```python
from build123d import *

# Parameters (mm, degrees)
F0_W     = 100
F0_H     = 100
F1_DEPTH = 15
F3_DEPTH = 25
F4_R     = 30
F5_DEPTH = 15.001
F6_W     = 20
F6_H     = 20
F7_DEPTH = 60
F8_W     = 80
F8_H     = 80
F9_DEPTH = 15.001


with BuildPart() as f1:
    # F0 (on Top) → F1 (new body)
    with BuildSketch(Plane.XY):
        Rectangle(F0_W, F0_H)
    extrude(amount=F1_DEPTH)

    # F2 (on face) → F3 (join)
    with BuildSketch(Plane.XY.offset(15)):
        Polygon((-30, -50), (-30, 30), (50, 30), (50, 50), (-50, 50), (-50, -50), align=None)
    extrude(amount=F3_DEPTH)

    # F4 (on face) → F5 (cut, through all)
    with BuildSketch(Plane.XY.offset(15)):
        with Locations((10, -10)):
            Circle(F4_R)
    extrude(amount=-F5_DEPTH, mode=Mode.SUBTRACT)

    # F6 (on face) → F7 (join)
    with BuildSketch(Plane.XY.offset(40)):
        with Locations((-40, 40)):
            Rectangle(F6_W, F6_H)
    extrude(amount=F7_DEPTH)

    # F8 (on face) → F9 (cut, through all)
    with BuildSketch(Plane.XY.offset(15)):
        with Locations((10, -10)):
            Rectangle(F8_W, F8_H)
    extrude(amount=-F9_DEPTH, mode=Mode.SUBTRACT)


solid = f1.part
```
Check sheet for the modelled part. Datum: model origin and axes. Units: mm. A direction names the side the tool comes from. Give positions to 0.01 mm unless a question says otherwise; leave off trailing zeros. Order: outer loops, then holes, each group sorted by start corner. A loop starts at its lowest first (then second) coordinate and runs counter-clockwise, first axis right, second up. Notation, with made-up numbers: M 31.5,30 L 70.5,30 A22 ccw 70.5,51 Z; hole C 3,55 d6. An arc over 180 degrees is marked long. Answer in a Markdown table with one row per item.
1) Access from +Z, -Z, +X, -X, +Y, -Y to the whole of each face (thin tool, end or side, straight path). Record for faces 1 (the flat face through (9, 40, 40)), 2 (the flat face through (-40, -9, 40)), 3 (the flat face through (-30, -11, 20)).
Filled sheet:
| item | result |
|---|---|
| face 1 | +Z, +X, +Y, -Y |
| face 2 | +Z, +X, -X, -Y |
| face 3 | +Z, -Z, +X, -Y |
2) Cross-section at D-D, the plane x = -22.5. Enter the section's corners in (y, z).
Filled sheet:
| item | result |
|---|---|
| outline | M 30,0 L 50,0 L 50,40 L 30,40 Z |
3) Cross-section at C-C, the plane z = 45.5. Enter the section's corners in (x, y), plus the area to 3 significant figures.
Filled sheet:
| item | result |
|---|---|
| outline | M -50,30 L -30,30 L -30,50 L -50,50 Z |
| area | 400 mm2 |
4) Gauge pin test, flat ends, axial feed: P1, Ø16, axis at x = -40.5, z = 84.5, coming from the -Y side; P2, Ø22, axis at x = -39, y = -5.5, coming from the +Z side; P3, Ø6, axis at y = 38.5, z = 64.5, coming from the +X side. Record the tip position at first contact, or that the pin passes through.
Filled sheet:
| item | result |
|---|---|
| P1 | stops at y = 30 |
| P2 | stops at z = 40 |
| P3 | stops at x = -30 |
5) Cross-section at B-B, the plane x = -39. Enter the section's corners in (y, z).
Filled sheet:
| item | result |
|---|---|
| outline | M -50,0 L 50,0 L 50,100 L 30,100 L 30,40 L -50,40 Z |
6) Thickness scan on L1, parallel to X at y = -31, z = 37.5; L2, parallel to Z at x = -38, y = -40.5; L3, parallel to Y at x = 40, z = 23. Record the ranges inside material, lowest first. Write a range as [from, to].
Filled sheet:
| item | result |
|---|---|
| L1 | x = [-50, -30] |
| L2 | z = [0, 40] |
| L3 | y = [30, 50] |
7) Cross-section at A-A, the plane y = 34.5. Enter the section's corners in (x, z), plus the area to 3 significant figures.
Filled sheet:
| item | result |
|---|---|
| outline | M -50,0 L 50,0 L 50,40 L -30,40 L -30,100 L -50,100 Z |
| area | 5,200 mm2 |
